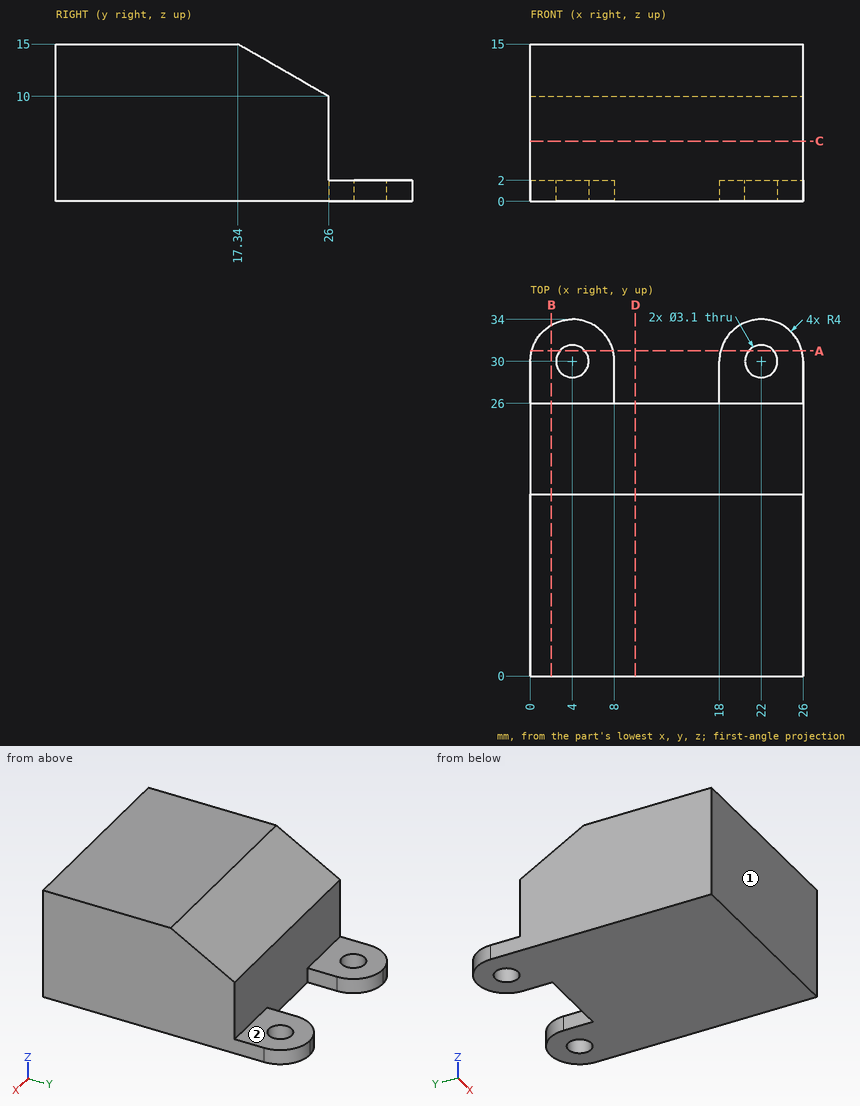
The figure shows three views and two pictorial views of one solid part (mm, origin at its lowest corner). Answer the questions. A direction names the side the tool comes from. Coordinates: 2 decimals unless noted, no trailing zeros. Loops run counter-clockwise (first coordinate to the right, second up) from the corner with the lowest first, then second, coordinate; pieces in that order, holes last. Notation, with made-up numbers: M -8,6 L -3,6 A19 cw -3,33 Z; hole C 67,83 d5. An arc over 180 degrees is marked long. Use CSV: the item, a comma, the result in double quotes. Start each with the question number.
(1) Find section C-C, the plane z = 5.75. Give the vertices of the cut face in (x, y).
(2) Find section A-A, the plane y = 31. Give the vertices of the cut face in (x, z).
(3) Find section B-B, the plane x = 2. Give the vertices of the cut face in (y, z).
(4) Consider line 1 (Y direction, x = 4, z = 1.55); line 2 (Y direction, x = 5, z = 8); line 3 (Y direction, x = 23.25, z = 12.75) (1 decimal). Determine where each line is inside the solid, lowest interval first.
(5) Find section D-D, the plane x = 10. Give the vertices of the cut face in (y, z).
(6) For the marked faces 1 and 2, determine the directions among +Z, -Z, +X, -X, +Y, -Y from which every point of the face is accessible in a straight line to the end or side of a thin tool.
(7) Given pin 1 Ø1 at (x, z) = (12.5, 5.5) entering from +Y; pin 2 Ø6.5 at (x, y) = (22, 31.5) entering from +Z, each flat-ended and moving along its own axis, determine where each tip first touches the part or whether it passes through.
Recorded:
1,outline,"M 0,0 L 26,0 L 26,26 L 0,26 Z"
2,outline,"M 0.13,0 L 2.82,0 L 2.82,2 L 0.13,2 Z; M 5.18,0 L 7.87,0 L 7.87,2 L 5.18,2 Z; M 18.13,0 L 20.82,0 L 20.82,2 L 18.13,2 Z; M 23.18,0 L 25.87,0 L 25.87,2 L 23.18,2 Z"
3,outline,"M 0,0 L 33.46,0 L 33.46,2 L 26,2 L 26,10 L 17.34,15 L 0,15 Z"
4,line 1,"y = 0 to 28.45, 31.55 to 34"
4,line 2,"y = 0 to 26"
4,line 3,"y = 0 to 21.2"
5,outline,"M 0,0 L 26,0 L 26,10 L 17.34,15 L 0,15 Z"
6,face 1,"+Z, -Z, +X, -X, -Y"
6,face 2,"+Z, +X, -X, +Y"
7,pin 1,"stops at y = 26"
7,pin 2,"stops at z = 2"
